from build123d import *

# Parameters (mm, degrees)
SKETCH_1_W          = 100
SKETCH_1_H          = 40
EXTRUDE_1_DEPTH     = 10
EXTRUDE_2_DEPTH     = 10
SKETCH_3_R          = 12.5
CUT_EXTRUDE_1_DEPTH = 5
SKETCH_7_R          = 6
CUT_EXTRUDE_2_DEPTH = 5
SKETCH_10_W         = 30
SKETCH_10_H         = 5
CUT_EXTRUDE_3_DEPTH = 85.409715081
SKETCH_14_R         = 4
CUT_EXTRUDE_4_DEPTH = 71.178344238
FILLET_2_R          = 8
FILLET_3_R          = 3


with BuildPart() as part:
    # Эскиз1 → Бобышка-Вытянуть1 (new body)
    with BuildSketch(Plane(origin=(0, 0, 0), x_dir=(1, 0, 0), z_dir=(0, 1, 0))):
        Rectangle(SKETCH_1_W, SKETCH_1_H)
    extrude(amount=EXTRUDE_1_DEPTH)

    # Эскиз2 → Бобышка-Вытянуть2 (add)
    with BuildSketch(Plane.XY.offset(20)):
        with BuildLine():
            Line((-20, 0), (-20, 35))
            ThreePointArc((-20, 35), (0, 55), (20, 35))
            Line((20, 35), (20, 0))
            Line((20, 0), (-20, 0))
        make_face()
    extrude(amount=-EXTRUDE_2_DEPTH)

    # Эскиз3 → Вырез-Вытянуть1 (cut)
    with BuildSketch(Plane.XY.offset(20)):
        with Locations((0, 35)):
            Circle(SKETCH_3_R)
    extrude(amount=-CUT_EXTRUDE_1_DEPTH, mode=Mode.SUBTRACT)

    # Эскиз7 → Вырез-Вытянуть2 (cut)
    with BuildSketch(Plane.XY.offset(15)):
        with Locations((0, 35)):
            Circle(SKETCH_7_R)
    extrude(amount=-CUT_EXTRUDE_2_DEPTH, mode=Mode.SUBTRACT)

    # Эскиз10 → Вырез-Вытянуть3 (cut, through all)
    with BuildSketch(Plane.XY.offset(20)):
        with Locations((0, 2.5)):
            Rectangle(SKETCH_10_W, SKETCH_10_H)
    extrude(amount=-CUT_EXTRUDE_3_DEPTH, mode=Mode.SUBTRACT)

    # Эскиз14 → Вырез-Вытянуть4 (cut, through all)
    with BuildSketch(Plane(origin=(0, 10, 0), x_dir=(1, 0, 0), z_dir=(0, 1, 0))):
        with Locations(Location((-42, 12, 0), (0, 0, 270))):
            Circle(SKETCH_14_R)
        with Locations(Location((42, 12, 0), (0, 0, 270))):
            Circle(SKETCH_14_R)
    extrude(amount=-CUT_EXTRUDE_4_DEPTH, mode=Mode.SUBTRACT)

    # Скругление2
    # the kernel refuses this fillet: 8 mm, written as the material it adds along each edge
    with BuildSketch(Plane(origin=(-15, 5, 20), x_dir=(0, -1, 0), z_dir=(0, 0, -1))) as fillet_2_piece_1:
        with BuildLine():
            CenterArc((8, -7.416198487), FILLET_2_R, 112.024312837, 67.975687163)
            Line((0, -7.416198487), (0, 0))
            Line((0, 0), (5, 0))
        make_face()
    extrude(amount=40)
    with BuildSketch(Plane(origin=(15, 5, 20), x_dir=(-1, 0, 0), z_dir=(0, 0, -1))) as fillet_2_piece_2:
        with BuildLine():
            CenterArc((7.416198487, -8), FILLET_2_R, 90, 67.975687163)
            Line((0, -5), (0, 0))
            Line((0, 0), (7.416198487, 0))
        make_face()
    extrude(amount=40)
    # the kernel refuses this fillet: 8 mm, written as the material it takes off along each edge
    with BuildSketch(Plane(origin=(50, -20, 20), x_dir=(-1, 0, 0), z_dir=(0, 1, 0)), Plane(origin=(50, -20, -20), x_dir=(0, 0, 1), z_dir=(0, 1, 0))) as fillet_2_2_piece_1:
        with BuildLine():
            CenterArc((FILLET_2_R, -FILLET_2_R), FILLET_2_R, 90, 90)
            Line((0, -FILLET_2_R), (0, 0))
            Line((0, 0), (FILLET_2_R, 0))
        make_face()
    extrude(amount=50, mode=Mode.SUBTRACT)
    with BuildSketch(Plane(origin=(-50, -20, 20), x_dir=(1, 0, 0), z_dir=(0, 1, 0)), Plane(origin=(-50, -20, -20), x_dir=(0, 0, 1), z_dir=(0, 1, 0))) as fillet_2_2_piece_2:
        with BuildLine():
            CenterArc((FILLET_2_R, FILLET_2_R), FILLET_2_R, 180, 90)
            Line((0, FILLET_2_R), (0, 0))
            Line((0, 0), (FILLET_2_R, 0))
        make_face()
    extrude(amount=50, mode=Mode.SUBTRACT)

    # Скругление3
    fillet_3_edges = [part.edges().sort_by_distance(p)[0] for p in [
        (31, 10, 20),
        (-20, 22.5, 20),
        (20, 22.5, 10),
        (-20, 22.5, 10),
        (0, 55, 10),
        (20, 22.5, 20),
        (0, 55, 20),
        (50, 10, 0),
        (-31, 10, 20),
        (0, 10, -20),
        (-50, 10, 0),
        (47.656854249, 10, -17.656854249),
        (-47.656854249, 10, -17.656854249),
        (-47.656854249, 10, 17.656854249),
        (47.656854249, 10, 17.656854249),
    ]]
    fillet(fillet_3_edges, radius=FILLET_3_R)


solid = part.part
Input: part model. Units: mm. Frame: model coordinates. A direction names the side the tool comes from. Coordinates: 2 decimals unless noted, no trailing zeros. Loops run counter-clockwise (first coordinate to the right, second up) from the corner with the lowest first, then second, coordinate; pieces in that order, holes last. Notation, with made-up numbers: (8, -19.5) -> (17, -19.5) arc R32 ccw to (17, 7.5) -> close; hole circle Ø2 at (-10, 11). An arc over 180 degrees is marked (long way). One line per item, written item: value.
(1) Set-up query: faces 1 (the face through (0, 5, 0)), 2 (the face through (-2.71, 22.797, 17.535)), 3 (the face through (-20, 22, 15)), 4 (the face through (29.68, 9.1, 19.14)). Return all of +Z, -Z, +X, -X, +Y, -Y with unobstructed straight access to the full face (end or side cutting, diameter ignored); none if empty.
Answer below:
face 1: +Z, -Z, -Y
face 2: +Z
face 3: +Z, -Z, -X, +Y
face 4: +Z, +X, +Y
(2) Cut plane A-A (x = 0). Output: boundary loops of the cut face in (y, z).
Answer below:
outline: (5, -20) -> (7, -20) arc R3 ccw to (10, -17) -> (10, 10) -> (29, 10) -> (29, 15) -> (22.5, 15) -> (22.5, 20) -> (5, 20) -> close; (41, 10) -> (52, 10) arc R3 ccw to (55, 13) -> (55, 17) arc R3 ccw to (52, 20) -> (47.5, 20) -> (47.5, 15) -> (41, 15) -> close
(3) Ray query, line 1 along X through (y, z) = (6, -12); line 2 along Y through (x, z) = (0, 13.7); line 3 along Y through (x, z) = (2, 1). Return the intervals inside material, ascending.
Answer below:
line 1: x = -50 to -46, -38 to 38, 46 to 50
line 2: y = 5 to 29, 41 to 55
line 3: y = 5 to 10
(4) Pin query (flat end, axial travel): pin 1 Ø8 at (x, y) = (12, 44) entering from -Z; pin 2 Ø4.5 at (y, z) = (22, 15) entering from +X; pin 3 Ø3 at (x, z) = (23, 5.5) entering from +Y; pin 4 Ø1 at (x, y) = (-21.5, 13.5) entering from -Z. Return the tip coordinate at first contact, or that it passes through.
Answer below:
pin 1: stops at z = 10
pin 2: stops at x = 20
pin 3: stops at y = 10
pin 4: passes through
(5) Cut plane B-B (z = 6.5). Output: boundary loops of the cut face in (x, y).
Answer below:
outline: (-50, 0) -> (-15, 0) arc R8 cw to (-7.58, 5) -> (7.58, 5) arc R8 cw to (15, 0) -> (50, 0) -> (50, 7) arc R3 ccw to (47, 10) -> (-47, 10) arc R3 ccw to (-50, 7) -> close
(6) Cut plane C-C (x = -23.5). Output: boundary loops of the cut face in (y, z), then the cut area to 3 significant figures.
Answer below:
outline: (0, -20) -> (7, -20) arc R3 ccw to (10, -17) -> (10, 17) arc R3 ccw to (7, 20) -> (0, 20) -> close
area: 396 mm2
(7) Draft query along X for faces 5 (the face through (19.1, 20.8, 19.14)), 6 (the face through (0, 55, 15)), 7 (the face through (-12.111, 3.596, 0.28)), 8 (the face through (-32, 0, 0)). Return one class per face: pulls with the +X half, pulls with the -X half, needs draft (parallel to the pull), parting line crosses it, or undercut.
Answer below:
face 5: pulls with the +X half
face 6: parting line crosses it
face 7: undercut
face 8: needs draft
(8) Cut plane D-D (x = 40.5). Output: boundary loops of the cut face in (y, z).
Answer below:
outline: (0, -20) -> (7, -20) arc R3 ccw to (10, -17) -> (10, -15.71) -> (0, -15.71) -> close; (0, -8.29) -> (10, -8.29) -> (10, 17) arc R3 ccw to (7, 20) -> (0, 20) -> close
